The model under review builds one solid part; all positions refer to its coordinate system, in mm. Face numbers are marked on the shaded views. A direction names the side the tool comes from. Give positions to 0.01 mm unless a question says otherwise; leave off trailing zeros. Loops run counter-clockwise (first coordinate to the right, second up) from the corner with the lowest first, then second, coordinate; pieces in that order, holes last. Notation, with made-up numbers: M 61.25,26 L 113.25,26 A14 cw 113.25,53 Z; hole C 53,12.25 d3. An arc over 180 degrees is marked long. Return JSON: item names as keys, results as strings. Group by question number.
```python
from build123d import *

# Parameters (mm, degrees)
F0_R      = 74.6125
F1_DEPTH  = 16.002
F2_R      = 49.2125
F3_DEPTH  = 58.674
F4_R      = 19.05
F5_DEPTH  = 74.677
F6_SIZE   = 1.27
F8_D      = 12.7
F8_DEPTH  = 19.05
F9_W      = 9.525
F9_H      = 27.94
F10_DEPTH = 74.677


with BuildPart() as f1:
    # F0 (on Top) → F1 (new body)
    with BuildSketch(Plane.XY):
        Circle(F0_R)
    extrude(amount=F1_DEPTH)

    # F2 (on face) → F3 (join)
    with BuildSketch(Plane(origin=(0, 0, 0), x_dir=(1, 0, 0), z_dir=(0, 0, -1))):
        Circle(F2_R)
    extrude(amount=F3_DEPTH)

    # F4 (on face) → F5 (cut, through all)
    with BuildSketch(Plane(origin=(0, 0, -58.674), x_dir=(1, 0, 0), z_dir=(0, 0, -1))):
        Circle(F4_R)
    extrude(amount=-F5_DEPTH, mode=Mode.SUBTRACT)

    # F6
    f6_edges = [f1.edges().sort_by_distance(p)[0] for p in [
        (-49.2125, 0, -58.674),
        (-74.6125, 0, 0),
        (-74.6125, 0, 16.002),
    ]]
    chamfer(f6_edges, length=F6_SIZE)

    # F8
    with Locations(Plane(origin=(0, 0, 0), x_dir=(1, 0, 0), z_dir=(0, 0, -1))):
        with Locations((-41.669327, 47.91573), (20.661576, 60.044561), (62.330903, 12.128831), (41.669327, -47.91573), (-20.661576, -60.044561), (-62.330903, -12.128831)):
            Hole(F8_D / 2, depth=F8_DEPTH)

    # F9 (on face) → F10 (cut, through all)
    with BuildSketch(Plane.XY.offset(16.002)):
        with Locations((0, -9.532987)):
            Rectangle(F9_W, F9_H)
    extrude(amount=-F10_DEPTH, mode=Mode.SUBTRACT)


solid = f1.part
```
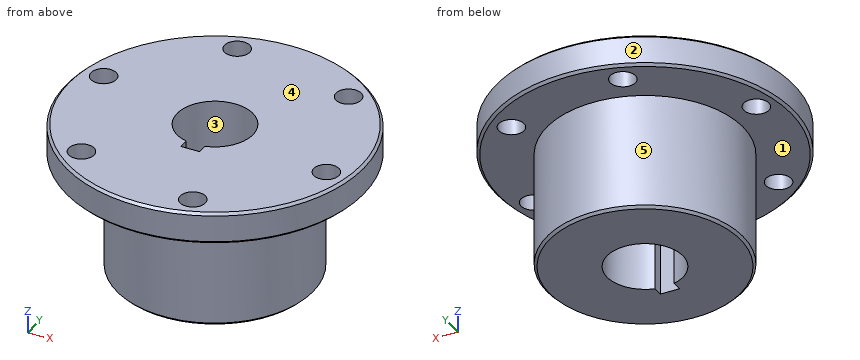
(1) For pin 1 (11.5 mm diameter, centred on x = 20.66, y = -60.04, fed in from +Z); pin 2 (4 mm diameter, centred on y = -20, z = -23.5, fed in from -X); pin 3 (3 mm diameter, centred on x = 0, z = -30, fed in from +Y); pin 4 (1 mm diameter, centred on x = -42.5, z = -33, fed in from -Y), all flat-tipped, find the tip position at first contact; note any pin that passes through.
(2) For the marked faces 4 and 5, list the 3-axis set-ups (+Z, -Z, +X, -X, +Y, -Y) from which the entire face can be reached by the end or side of a thin tool; tool diameter is ignored.
(3) Add section A-A (y = 0). Write out the cut boundary in (x, z), and give its area (3 significant figures).
(4) For probe 1 along Y at (x, z) = (-1, -13); probe 2 along X at (y, z) = (0, -36); probe 3 along Z at (x, y) = (-63, -9), list the stretches that pass through material, from the lowest coordinate up.
(5) Add section B-B (x = 0). Write out the cut boundary in (y, z).
(6) Mouldability with a two-part tool opening along X and no side actions: class the marked faces 1, 2 and 3 as released by +X, released by -X, zero draft, split by the parting line, or undercut.
(7) Add section D-D (y = -16). Count the separate pieces of the cut face and the enclosed holes in it, and give its area (3 significant figures).
Verdict:
{
 "1": {"pin 1": "passes through", "pin 2": "stops at x = -45.8", "pin 3": "stops at y = 49.21", "pin 4": "stops at y = -25.65"},
 "2": {"face 4": "+Z, +X, -X, +Y, -Y", "face 5": "-Z"},
 "3": {"outline": "M -74.61,1.27 L -73.34,0 L -49.21,0 L -49.21,-57.4 L -47.94,-58.67 L -19.05,-58.67 L -19.05,16 L -73.34,16 L -74.61,14.73 Z; M 19.05,-58.67 L 47.94,-58.67 L 49.21,-57.4 L 49.21,0 L 73.34,0 L 74.61,1.27 L 74.61,14.73 L 73.34,16 L 19.05,16 Z", "area": "5,310 mm²"},
 "4": {"probe 1": "y = -49.2 to -23.5, 19.02 to 49.2", "probe 2": "x = -49.21 to -19.05, 19.05 to 49.21", "probe 3": "z = 0 to 16"},
 "5": {"outline": "M -74.61,1.27 L -73.34,0 L -49.21,0 L -49.21,-57.4 L -47.94,-58.67 L -23.5,-58.67 L -23.5,16 L -73.34,16 L -74.61,14.73 Z; M 19.05,-58.67 L 47.94,-58.67 L 49.21,-57.4 L 49.21,0 L 73.34,0 L 74.61,1.27 L 74.61,14.73 L 73.34,16 L 19.05,16 Z"},
 "6": {"face 1": "zero draft", "face 2": "split by the parting line", "face 3": "undercut"},
 "7": {"separate pieces": "3", "enclosed holes": "0", "area": "6,080 mm²"}
}
